For this review, take the finished solid that the model builds, in its own axes (mm). A direction names the side the tool comes from. Give positions to 0.01 mm unless a question says otherwise; leave off trailing zeros. Loops run counter-clockwise (first coordinate to the right, second up) from the corner with the lowest first, then second, coordinate; pieces in that order, holes last. Notation, with made-up numbers: (9, 41) - (51, 41) arc R21 cw to (51, 55) - close; hole circle Ø4 at (-33, -38.5). An arc over 180 degrees is marked (long way). Put each result on its own line as item: value. Start each with the question number.
from build123d import *

# Parameters (mm, degrees)
SKETCH1_W           = 134.5
SKETCH1_H           = 157
SKETCH1_R           = 2.1
SKETCH1_W_2         = 118
SKETCH1_H_2         = 119.8
BOSS_EXTRUDE1_DEPTH = 5
CUT_EXTRUDE1_START  = -1.57
SKETCH2_W           = 90.947883714
SKETCH2_H           = 6.05
CUT_EXTRUDE1_DEPTH  = 1.57
SKETCH3_W           = 90.9
SKETCH3_H           = 11.55
BOSS_EXTRUDE2_DEPTH = 6
SKETCH4_W           = 120.05
SKETCH4_H           = 121.85
CUT_EXTRUDE2_DEPTH  = 1.65


with BuildPart() as part:
    # Sketch1 → Boss-Extrude1 (new body)
    with BuildSketch(Plane.XY.offset(6.1)):
        Rectangle(SKETCH1_W, SKETCH1_H)
        with Locations((-48.05, 70.990439644)):
            Circle(SKETCH1_R, mode=Mode.SUBTRACT)
        with Locations((48.05, 70.990439644)):
            Circle(SKETCH1_R, mode=Mode.SUBTRACT)
        with Locations((48.05, -70.990439644)):
            Circle(SKETCH1_R, mode=Mode.SUBTRACT)
        with Locations((-48.05, -70.990439644)):
            Circle(SKETCH1_R, mode=Mode.SUBTRACT)
        Rectangle(SKETCH1_W_2, SKETCH1_H_2, mode=Mode.SUBTRACT)
    extrude(amount=BOSS_EXTRUDE1_DEPTH)

    # Sketch2 → Cut-Extrude1 (cut)
    with BuildSketch(Plane(origin=(0, 0, 6.1), x_dir=(-1, 0, 0), z_dir=(0, 0, -1)).offset(CUT_EXTRUDE1_START)):
        with Locations((0.001058143, 63.925)):
            Rectangle(SKETCH2_W, SKETCH2_H)
        with Locations((0.001058143, -63.925)):
            Rectangle(SKETCH2_W, SKETCH2_H)
    extrude(amount=CUT_EXTRUDE1_DEPTH, mode=Mode.SUBTRACT)

    # Sketch3 → Boss-Extrude2 (add)
    with BuildSketch(Plane.XY.offset(0.1)):
        with Locations((0, -72.725)):
            Rectangle(SKETCH3_W, SKETCH3_H)
        with Locations((0, 72.725)):
            Rectangle(SKETCH3_W, SKETCH3_H)
    extrude(amount=BOSS_EXTRUDE2_DEPTH)

    # Sketch4 → Cut-Extrude2 (cut)
    with BuildSketch(Plane(origin=(0, 0, 6.1), x_dir=(-1, 0, 0), z_dir=(0, 0, -1))):
        Rectangle(SKETCH4_W, SKETCH4_H)
    extrude(amount=-CUT_EXTRUDE2_DEPTH, mode=Mode.SUBTRACT)


solid = part.part
1) Take a section at A-A on x = -53. State the section outline as (y, z) points (3 decimals).
2) Wall thickness on probe 1 along Y at (x, z) = (-48.05, 8.3); probe 2 along X at (y, z) = (37.5, 10.5); probe 3 along Y at (x, z) = (-2, 5.75): over which ranges is each line inside the solid? List them lowest first.
3) Take a section at C-C on x = 48.05. State the section outline as (y, z) points (3 decimals).
4) Machinability: for faces 1 (the flat face through (45.45, -73, 3)), 2 (the flat face through (1, -66.95, 4)), 3 (the flat face through (-59, -1, 9)), 4 (the flat face through (-61, 1, 6.1)), which of the approach directions +Z, -Z, +X, -X, +Y, -Y give a long, thin tool a straight path to every point of the face, cutting with its end or side? Answer none if there is none.
5) Take a section at B-B on y = -45.5. State the section outline as (x, z) points (3 decimals), and give its area (3 significant figures).
6) Insertion check: P1, Ø1.8, axis at x = 10.5, y = -64, coming from the -Z side. The pin has a flat end and moves straight along its axis. Give the tip position at first contact, or say it passes through.
7) Take a section at D-D on x = -17.5. State the section outline as (y, z) points (3 decimals), and give its area (3 significant figures).
Answers follow:
1. outline: (-78.5, 6.1) - (-60.925, 6.1) - (-60.925, 7.75) - (-59.9, 7.75) - (-59.9, 11.1) - (-78.5, 11.1) - close; (59.9, 7.75) - (60.925, 7.75) - (60.925, 6.1) - (78.5, 6.1) - (78.5, 11.1) - (59.9, 11.1) - close
2. probe 1: -78.5 to -73.09, -68.89 to -59.9, 59.9 to 68.89, 73.09 to 78.5
2. probe 2: -67.25 to -59, 59 to 67.25
2. probe 3: -78.5 to -66.95, 66.95 to 78.5
3. outline: (-78.5, 6.1) - (-73.09, 6.1) - (-73.09, 11.1) - (-78.5, 11.1) - close; (-68.89, 6.1) - (-60.925, 6.1) - (-60.925, 7.75) - (-59.9, 7.75) - (-59.9, 11.1) - (-68.89, 11.1) - close; (59.9, 7.75) - (60.925, 7.75) - (60.925, 6.1) - (68.89, 6.1) - (68.89, 11.1) - (59.9, 11.1) - close; (73.09, 6.1) - (78.5, 6.1) - (78.5, 11.1) - (73.09, 11.1) - close
4. face 1: -Z, +X, +Y, -Y
4. face 2: -Z
4. face 3: +Z, -Z
4. face 4: -Z, -X, +Y, -Y
5. outline: (-67.25, 6.1) - (-60.025, 6.1) - (-60.025, 7.75) - (-59, 7.75) - (-59, 11.1) - (-67.25, 11.1) - close; (59, 7.75) - (60.025, 7.75) - (60.025, 6.1) - (67.25, 6.1) - (67.25, 11.1) - (59, 11.1) - close
5. area: 79.1 mm2
6. P1: z = 7.67
7. outline: (-78.5, 0.1) - (-66.95, 0.1) - (-66.95, 7.67) - (-60.925, 7.67) - (-60.925, 7.75) - (-59.9, 7.75) - (-59.9, 11.1) - (-78.5, 11.1) - close; (59.9, 7.75) - (60.925, 7.75) - (60.925, 7.67) - (66.95, 7.67) - (66.95, 0.1) - (78.5, 0.1) - (78.5, 11.1) - (59.9, 11.1) - close
7. area: 302 mm2
